from build123d import *

# Parameters (mm, degrees)
F1_DEPTH = 80
F2_W     = 32.294086
F2_H     = 10.712334
F3_DEPTH = 15
F4_W     = 13.147677
F4_H     = 28.905093
F5_DEPTH = 25


with BuildPart() as f1:
    # F0 (on Front) → F1 (new body)
    with BuildSketch(Plane.XZ):
        Polygon((-22.541075, 39.326958), (-33.147677, 28.720356), (-33.147677, -41.279644), (-22.541075, -51.886245), (-22.541075, -66.886245), (-2.541075, -86.886245), (-2.541075, -66.886245), (-13.147677, -56.279644), (-13.147677, 43.720356), (-2.541075, 54.326958), (-2.541075, 74.326958), (-22.541075, 54.326958), align=None)
    extrude(amount=F1_DEPTH)

    # F2 (on face) → F3 (join)
    with BuildSketch(Plane.YZ.offset(-13.147677)):
        with Locations((-40, 0)):
            Rectangle(F2_W, F2_H)
    extrude(amount=F3_DEPTH)

    # F4 (on face) → F5 (cut)
    with BuildSketch(Plane.XY.offset(5.356167)):
        with Locations((-6.573838, -40.174481)):
            Rectangle(F4_W, F4_H)
    extrude(amount=-F5_DEPTH, mode=Mode.SUBTRACT)


solid = f1.part
Input: part model. Units: mm. Frame: model coordinates. A direction names the side the tool comes from. Give positions to 0.01 mm unless a question says otherwise; leave off trailing zeros. Loops run counter-clockwise (first coordinate to the right, second up) from the corner with the lowest first, then second, coordinate; pieces in that order, holes last. Notation, with made-up numbers: M 17,29.25 L 34,29.25 A23 ccw 34,37.25 Z; hole C 18.25,86.25 d8. An arc over 180 degrees is marked long. Use one line per item in the form item = value.
1. Section query D-D, the plane z = -39. Return the cut outline in (x, y).
Numbers:
outline = M -33.15,-80 L -13.15,-80 L -13.15,0 L -33.15,0 Z
2. Line query: L1, parallel to Z at x = -8, y = -68.5; L2, parallel to Z at x = -3, y = -36; L3, parallel to X at y = -13, z = -28. Output: solid intervals per line, ascending.
Numbers:
L1 = -81.43 to -61.43, 48.87 to 68.87
L2 = -86.43 to -66.43, 53.87 to 73.87
L3 = -33.15 to -13.15
3. First-contact query: pin 1 (7.5 mm diameter, centred on y = -39, z = 45, fed in from -X); pin 2 (6 mm diameter, centred on y = -41, z = 66.5, fed in from +X); pin 3 (2 mm diameter, centred on y = -38, z = 18.5, fed in from +X); pin 4 (1 mm diameter, centred on x = -11.5, z = -24, fed in from +Y). Flat tips, straight axial feed; report the tip coordinate or a pass-through.
Numbers:
pin_1 = -22.54
pin_2 = -2.54
pin_3 = -13.15
pin_4 = through
4. Section query B-B, the plane x = -8.5. Return the cut outline in (y, z).
Numbers:
outline = M -80,-80.93 L 0,-80.93 L 0,-60.93 L -80,-60.93 Z; M -80,48.37 L 0,48.37 L 0,68.37 L -80,68.37 Z; M -56.15,-5.36 L -54.63,-5.36 L -54.63,5.36 L -56.15,5.36 Z; M -25.72,-5.36 L -23.85,-5.36 L -23.85,5.36 L -25.72,5.36 Z
5. Reachability of faces 1 (the face through (1, -40, 5.356)), 2 (the face through (-7, -54.627, 0)), 3 (the face through (-18, 0, -5)), 4 (the face through (-22.541, -39, -59)) from +Z, -Z, +X, -X, +Y, -Y: full face, straight path, thin tool, end or side. Return the list, or none.
Numbers:
face_1 = +X, +Y, -Y
face_2 = none
face_3 = +Z, -Z, +X, -X, +Y
face_4 = -Z, -X, +Y, -Y
6. Pull-direction query (Z, two-part tool) for faces 5 (the face through (-7.92, -39.44, 48.95)), 6 (the face through (-12.4, -39.44, 64.47)), 7 (the face through (-22.541, -39, 47)); classes: released by +Z, released by -Z, zero draft, split by the parting line, or undercut.
Numbers:
face_5 = undercut
face_6 = released by +Z
face_7 = zero draft
7. Section query A-A, the plane y = -43.5. Return the cut outline in (x, z).
Numbers:
outline = M -33.15,-41.28 L -22.54,-51.89 L -22.54,-66.89 L -2.54,-86.89 L -2.54,-66.89 L -13.15,-56.28 L -13.15,43.72 L -2.54,54.33 L -2.54,74.33 L -22.54,54.33 L -22.54,39.33 L -33.15,28.72 Z; M 0,-5.36 L 1.85,-5.36 L 1.85,5.36 L 0,5.36 Z
8. Section query C-C, the plane y = -74.5. Return the cut outline in (x, z).
Numbers:
outline = M -33.15,-41.28 L -22.54,-51.89 L -22.54,-66.89 L -2.54,-86.89 L -2.54,-66.89 L -13.15,-56.28 L -13.15,43.72 L -2.54,54.33 L -2.54,74.33 L -22.54,54.33 L -22.54,39.33 L -33.15,28.72 Z
